Could you check a few things on this model? Use its own coordinates, in mm. Give positions to 0.01 mm unless a question says otherwise; leave off trailing zeros. Write each loop counter-clockwise with the first axis right and the second up, starting at its lowest first coordinate (ties: lowest second). Pieces come first, ordered by that corner, then holes. Notation, with made-up numbers: (36.25, 63) - (76.25, 63) arc R16 cw to (76.25, 77) - close; hole circle Ø5 at (81.25, 70.25). An arc over 180 degrees is marked (long way). Answer as a JSON object with one key per item and string values. Group by question number.
```python
from build123d import *

# Parameters (mm, degrees)
SKETCH_1_W        = 60
SKETCH_1_H        = 60
EXTRUDE_1_DEPTH   = 2
CHAMFER_1_SIZE    = 2
HOLE_WIZARD_M61_D = 6.6


with BuildPart() as part:
    # Эскиз1 → Бобышка-Вытянуть1 (new body)
    with BuildSketch(Plane.XY):
        Rectangle(SKETCH_1_W, SKETCH_1_H)
    extrude(amount=EXTRUDE_1_DEPTH)

    # Фаска1
    chamfer_1_edges = [part.edges().sort_by_distance(p)[0] for p in [
        (30, -30, 1),
        (-30, -30, 1),
        (-30, 30, 1),
        (30, 30, 1),
    ]]
    chamfer(chamfer_1_edges, length=CHAMFER_1_SIZE)

    # Отверстие с зазором M61 (through all)
    with Locations(Plane.XY.offset(2)):
        with Locations((-15, 15), (15, 15), (-15, -15), (15, -15), (-15, 45), (15, 45), (15, -45), (-15, -45)):
            Hole(HOLE_WIZARD_M61_D / 2)


solid = part.part
```
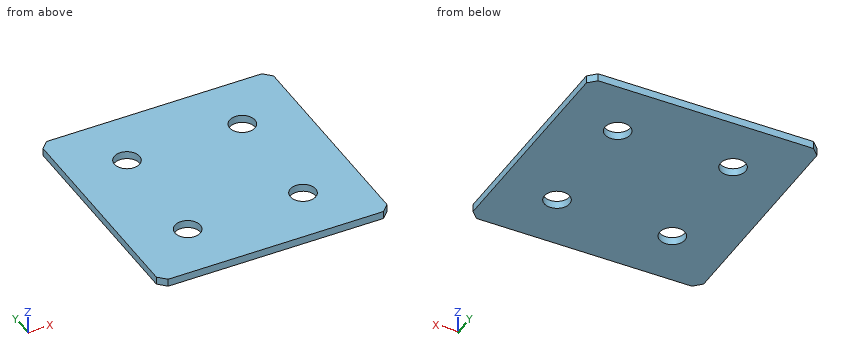
(1) I want a section at A-A, the plane y = 15. Please give me the cut outline in (x, z).
(2) I want a section at B-B, the plane z = 0.95. Please give me the cut outline in (x, y), and give its area (3 significant figures).
(3) I need wall thicknesses on L1, parallel to Y at x = 15, z = 0.65; L2, parallel to X at y = -14.5, z = 0.3; L3, parallel to X at y = 12.5, z = 0.4. Which ranges of each line are inside material? Lowest first, please.
Entries:
{
 "1": {"outline": "(-30, 0) - (-18.3, 0) - (-18.3, 2) - (-30, 2) - close; (-11.7, 0) - (11.7, 0) - (11.7, 2) - (-11.7, 2) - close; (18.3, 0) - (30, 0) - (30, 2) - (18.3, 2) - close"},
 "2": {"outline": "(-30, -28) - (-28, -30) - (28, -30) - (30, -28) - (30, 28) - (28, 30) - (-28, 30) - (-30, 28) - close; hole circle Ø6.6 at (-15, -15); hole circle Ø6.6 at (-15, 15); hole circle Ø6.6 at (15, -15); hole circle Ø6.6 at (15, 15)", "area": "3,460 mm^2"},
 "3": {"L1": "-30 to -18.3, -11.7 to 11.7, 18.3 to 30", "L2": "-30 to -18.26, -11.74 to 11.74, 18.26 to 30", "L3": "-30 to -17.15, -12.85 to 12.85, 17.15 to 30"}
}
